Build history of the part. All positions in model axes, mm. A direction names the side the tool comes from. Round coordinates to 2 decimals unless told otherwise and drop trailing zeros. Write each loop counter-clockwise with the first axis right and the second up, starting at its lowest first coordinate (ties: lowest second). Pieces come first, ordered by that corner, then holes.
from build123d import *

# Parameters (mm, degrees)
BOSS_EXTRUDE1_DEPTH = 1
SKETCH2_R           = 2.5
SKETCH2_R_2         = 1.5
BOSS_EXTRUDE2_DEPTH = 1
SKETCH2_2_R         = 1.5
BOSS_EXTRUDE3_DEPTH = 6
FILLET1_R           = 2


with BuildPart() as part:
    # Sketch1 → Boss-Extrude1 (new, symmetric)
    with BuildSketch(Plane(origin=(0, 0, 0), x_dir=(1, 0, 0), z_dir=(0, 1, 0))):
        with BuildLine():
            Line((0, -7.166621556), (0, 7.166621556))
            ThreePointArc((0, 7.166621556), (-0.554836306, 8.90477417), (-2.01411634, 10))
            ThreePointArc((-2.01411634, 10), (-19.83571516, 14.416393561), (-38.164373421, 15.5))
            ThreePointArc((-38.164373421, 15.5), (-41.593178753, 13.979636076), (-43, 10.502702593))
            Line((-43, 10.502702593), (-43, -10.502702593))
            ThreePointArc((-43, -10.502702593), (-41.593178753, -13.979636076), (-38.164373421, -15.5))
            ThreePointArc((-38.164373421, -15.5), (-19.83571516, -14.416393561), (-2.01411634, -10))
            ThreePointArc((-2.01411634, -10), (-0.554836306, -8.90477417), (0, -7.166621556))
        make_face()
    extrude(amount=BOSS_EXTRUDE1_DEPTH, both=True)

    # Sketch2 → Boss-Extrude2 (add)
    with BuildSketch(Plane.XZ.offset(1)):
        with Locations(Location((-8, 0, 0), (0, 0, 270))):
            Circle(SKETCH2_R)
        with Locations(Location((-8, 0, 0), (0, 0, 270))):
            Circle(SKETCH2_R_2, mode=Mode.SUBTRACT)
    boss_extrude2 = extrude(amount=BOSS_EXTRUDE2_DEPTH)

    # Sketch2<2> → Boss-Extrude3 (add)
    with BuildSketch(Plane.XZ.offset(1)):
        with Locations(Location((-8, 0, 0), (0, 0, 270))):
            Circle(SKETCH2_2_R)
    boss_extrude3 = extrude(amount=BOSS_EXTRUDE3_DEPTH)

    # Sketch-Pattern1: Boss-Extrude2, Boss-Extrude3 at 2 more places
    with Locations((-30, 0, 10.502703), (-30, 0, -10.502703)):
        add(boss_extrude2)
        add(boss_extrude3)

    # Fillet1
    fillet1_edges = [part.edges().sort_by_distance(p)[0] for p in [
        (-19.83571516, 1, 14.416393561),
        (-41.593178753, 1, 13.979636076),
        (-43, 1, 0),
        (-41.593178753, 1, -13.979636076),
        (-0.554836306, 1, -8.90477417),
        (0, 1, 0),
        (-0.554836306, 1, 8.90477417),
        (-19.83571516, 1, -14.416393561),
    ]]
    fillet(fillet1_edges, radius=FILLET1_R - 0.0001)  # a hair under: the kernel refuses the full size


solid = part.part
1) Slice it at B-B (y = -1.5). Write the cut outline in (x, z), plus the area to 3 significant figures.
Results:
outline: circle Ø5 at (-38, -10.5); circle Ø5 at (-38, 10.5); circle Ø5 at (-8, 0)
area: 58.9 mm2
2) Mould opens along Z. For faces 3 (the flat face through (-38, -7, -10)), 4 (the cylindrical face through (-40.44, -1.49, -9.96)), 5 (the cylindrical face through (-9.464, -4.465, 0.325)), 6 (the flat face through (-39, -2, -12)) say: released by +Z, released by -Z, zero draft, split by the parting line, or undercut.
Results:
face 3: zero draft
face 4: undercut
face 5: split by the parting line
face 6: undercut
3) Which spindle directions (+Z, -Z, +X, -X, +Y, -Y) get a long thin tool onto all of the face, cutting with end or side? Do faces 1 (the flat face through (-10, -2, 0)), 2 (the cylindrical face through (-0.57, 0.4, -0.1)). Say none if no direction does.
Results:
face 1: -Y
face 2: +Z, -Z, +X, +Y
4) Wall check: L1, parallel to Z at x = -36, y = -1.5; L2, parallel to Y at x = -29.5, z = 13.5; L3, parallel to X at y = -3.75, z = -1. Give the ranges that are in metal, low to high.
Results:
L1: z = -12 to -9, 9 to 12
L2: y = -1 to 1
L3: x = -9.12 to -6.88
5) Slice it at C-C (y = -4.5). Write the cut outline in (x, z).
Results:
outline: circle Ø3 at (-38, -10.5); circle Ø3 at (-38, 10.5); circle Ø3 at (-8, 0)
6) Pin check, flat tips, straight feed: pin 1 Ø5 at (x, z) = (-19, -4) entering from -Y; pin 2 Ø1 at (y, z) = (-2.5, -4) entering from -X; pin 3 Ø1.5 at (x, y) = (-14, -0.5) entering from +Z; pin 4 Ø5 at (x, z) = (-33.5, 9.5) entering from -Y. Stop position of each tip, or through.
Results:
pin 1: stops at y = -1
pin 2: passes through
pin 3: stops at z = 13.48
pin 4: stops at y = -2
